```python
from build123d import *

# Parameters (mm, degrees)
SKETCH5_W           = 20
SKETCH5_H           = 20
BOSS_EXTRUDE1_DEPTH = 40
SKETCH7_W           = 12
SKETCH7_H           = 5.480254557
CUT_EXTRUDE3_DEPTH  = 20
SKETCH8_W           = 10
SKETCH8_H           = 10
CUT_EXTRUDE5_DEPTH  = 20
SKETCH12_R          = 3
CUT_EXTRUDE9_DEPTH  = 20
SKETCH16_R          = 4
CUT_EXTRUDE10_DEPTH = 2.5
CUT_EXTRUDE11_START = -2.5
SKETCH17_R          = 4
CUT_EXTRUDE11_DEPTH = 2.5
FILLET8_R           = 8
SKETCH18_R          = 6.023611462
BOSS_EXTRUDE2_DEPTH = 3
SKETCH19_R          = 4
CUT_EXTRUDE12_DEPTH = 10


with BuildPart() as part:
    # Sketch5 → Boss-Extrude1 (new body)
    with BuildSketch(Plane.XY):
        with Locations((0.782482396, -0.960509114)):
            Rectangle(SKETCH5_W, SKETCH5_H)
    extrude(amount=BOSS_EXTRUDE1_DEPTH)

    # Sketch7 → Cut-Extrude3 (cut)
    with BuildSketch(Plane(origin=(10.782482396, 0, 0), x_dir=(0, 0, -1), z_dir=(1, 0, 0))):
        Polygon((-40, 9.039490886), (-40, -0.960509114), (-22, 9.039490886), align=None)
        with Locations((-16, -8.220381835)):
            Rectangle(SKETCH7_W, SKETCH7_H)
        Polygon((-10, 9.039490886), (0, -2.740127279), (0, 9.039490886), align=None)
    extrude(amount=-CUT_EXTRUDE3_DEPTH, mode=Mode.SUBTRACT)

    # Sketch8 → Cut-Extrude5 (cut)
    with BuildSketch(Plane.XZ.offset(10.960509114)):
        with BuildLine():
            Line((-9.217517604, 0), (0.78248238, 0))
            ThreePointArc((0.78248238, 0), (-6.288585421, 2.928932194), (-9.217517604, 10))
            Line((-9.217517604, 10), (-9.217517604, 0))
        make_face()
        with BuildLine():
            Line((10.782482396, 0), (10.782482396, 10))
            ThreePointArc((10.782482396, 10), (7.853550202, 2.928932182), (0.78248238, 0))
            Line((0.78248238, 0), (10.782482396, 0))
        make_face()
        with Locations((0.782482396, 35)):
            Rectangle(SKETCH8_W, SKETCH8_H)
    extrude(amount=-CUT_EXTRUDE5_DEPTH, mode=Mode.SUBTRACT)

    # Sketch10 → Cut-Revolve2 (revolve, cut)
    with BuildSketch(Plane(origin=(0, 9.039490886, 0), x_dir=(1, 0, 0), z_dir=(0, 1, 0))):
        with BuildLine():
            Line((-5.217517604, -16), (6.782482396, -16))
            ThreePointArc((6.782482396, -16), (0.782482396, -22), (-5.217517604, -16))
        make_face()
    revolve(axis=Axis((-5.217517604, 9.039490886, 16), (1, 0, 0)), mode=Mode.SUBTRACT)

    # Sketch12 → Cut-Extrude9 (cut)
    with BuildSketch(Plane(origin=(10.782482396, 0, 0), x_dir=(0, 0, -1), z_dir=(1, 0, 0))):
        with Locations(Location((-35, -5.960509114, 0), (0, 0, 90))):
            Circle(SKETCH12_R)
    extrude(amount=-CUT_EXTRUDE9_DEPTH, mode=Mode.SUBTRACT)

    # Sketch16 → Cut-Extrude10 (cut)
    with BuildSketch(Plane(origin=(10.782482396, 0, 0), x_dir=(0, 0, -1), z_dir=(1, 0, 0))):
        with Locations(Location((-35, -5.960509114, 0), (0, 0, 90))):
            Circle(SKETCH16_R)
    extrude(amount=-CUT_EXTRUDE10_DEPTH, mode=Mode.SUBTRACT)

    # Sketch17 → Cut-Extrude11 (cut)
    with BuildSketch(Plane.ZY.offset(9.217517604).offset(CUT_EXTRUDE11_START)):
        with Locations(Location((35, -5.960509114, 0), (0, 0, 90))):
            Circle(SKETCH17_R)
    extrude(amount=CUT_EXTRUDE11_DEPTH, mode=Mode.SUBTRACT)

    # Fillet8
    fillet8_edges = [part.edges().sort_by_distance(p)[0] for p in [
        (-6.717517604, -0.960509114, 40),
        (8.282482396, -0.960509114, 40),
    ]]
    fillet(fillet8_edges, radius=FILLET8_R)

    # Sketch18 → Boss-Extrude2 (add)
    with BuildSketch(Plane(origin=(0, -5.480254557, 0), x_dir=(-1, 0, 0), z_dir=(0, -1, 0))):
        with Locations((-0.782482396, -16)):
            Circle(SKETCH18_R)
    extrude(amount=BOSS_EXTRUDE2_DEPTH)

    # Sketch19 → Cut-Extrude12 (cut)
    with BuildSketch(Plane(origin=(0, -8.480254557, 0), x_dir=(-1, 0, 0), z_dir=(0, -1, 0))):
        with Locations(Location((-0.782482396, -16, 0), (0, 0, 180))):
            Circle(SKETCH19_R)
    extrude(amount=-CUT_EXTRUDE12_DEPTH, mode=Mode.SUBTRACT)


solid = part.part
```
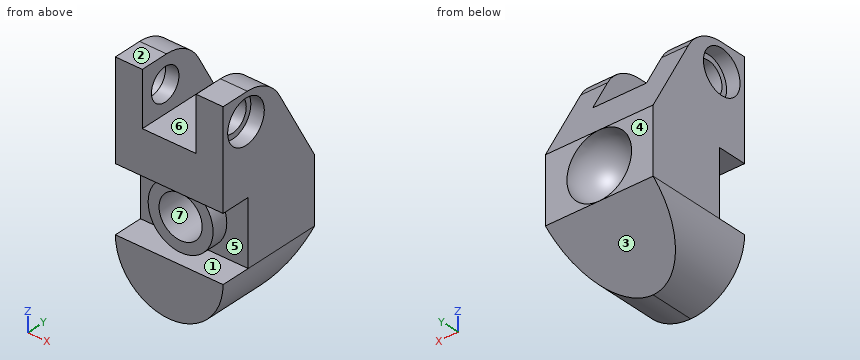
Here's how the part is built. I have some questions about the finished solid (model axes, mm). Face numbers are marked on the shaded views. A direction names the side the tool comes from. Give positions to 0.01 mm unless a question says otherwise; leave off trailing zeros. Loops run counter-clockwise (first coordinate to the right, second up) from the corner with the lowest first, then second, coordinate; pieces in that order, holes last. Notation, with made-up numbers: M 28.5,51 L 54.5,51 A25 ccw 54.5,81 Z; hole C -11.75,33.5 d1. An arc over 180 degrees is marked long. Put each result on its own line as item: value. Start each with the question number.
(1) I want a section at D-D on z = 16. Please give me the cut outline in (x, y), then the cut area to 3 significant figures.
(2) I want a section at B-B on y = 6.5. Please give me the cut outline in (x, z), then the cut area to 3 significant figures.
(3) I want a section at A-A on x = 7.25. Please give me the cut outline in (y, z).
(4) I need wall thicknesses on line 1 along X through (y, z) = (-1.75, 32.5); line 2 along X through (y, z) = (5, 12.5); line 3 along Y through (x, z) = (-4.25, 30). Which ranges of each line are inside material? Lowest first, please. Write a range as [from, to].
(5) If we mould it in two halves opening along Z, with no side actions, what happens to the marked faces 1, 2, 3 and 4? For each: +Z half, -Z half, draft (parallel to the pull), parting line (faces both ways), or undercut.
(6) I want a section at C-C on z = 35. Please give me the cut outline in (x, y), then the cut area to 3 significant figures.
(7) Will these pins go through, and if not, where does the flat tip stop? pin 1 Ø5.5 at (y, z) = (-5.96, 35) entering from +X; pin 2 Ø7 at (x, z) = (0.78, 16) entering from -Y; pin 3 Ø6.5 at (x, z) = (0.5, 17.5) entering from -Y; pin 4 Ø2 at (x, y) = (0.5, 4) entering from -Z.
(8) For the marked faces 5, 6 and 7, which set-ups out of +Z, -Z, +X, -X, +Y, -Y let a thin tool reach every point of the face, with its end or its side?
Answer block:
1. outline: M -9.22,-5.48 L -5.24,-5.48 L -5.24,-8.48 L -3.22,-8.48 L -3.22,1.52 L 4.78,1.52 L 4.78,-8.48 L 6.81,-8.48 L 6.81,-5.48 L 10.78,-5.48 L 10.78,9.04 L 6.78,9.04 A6 cw -5.22,9.04 L -9.22,9.04 Z
1. area: 190 mm^2
2. outline: M -9.22,10 A10 ccw -8.98,7.84 L 10.55,7.84 A10 ccw 10.78,10 L 10.78,26.57 L -9.22,26.57 Z; hole C 0.78,16 d10.87
2. area: 281 mm^2
3. outline: M -10.96,2.37 L 0.06,2.37 L 9.04,10 L 9.04,22 L 1.33,35.89 A8 ccw -5.67,40 L -10.96,40 L -10.96,22 L -5.48,22 L -5.48,10 L -10.96,10 Z; hole C -5.96,35 d6
4. line 1: [-9.22, -4.22], [5.78, 10.78]
4. line 2: [-9.22, -1.94], [3.51, 10.78]
4. line 3: [-10.96, 4.6]
5. face 1: undercut
5. face 2: +Z half
5. face 3: -Z half
5. face 4: draft
6. outline: M -9.22,-10.96 L -4.22,-10.96 L -4.22,-8.96 L -6.72,-8.96 L -6.72,-9.96 L -9.22,-9.96 Z; M -9.22,-1.96 L -6.72,-1.96 L -6.72,-2.96 L -4.22,-2.96 L -4.22,1.82 L -9.22,1.82 Z; M 5.78,-10.96 L 10.78,-10.96 L 10.78,-9.96 L 8.28,-9.96 L 8.28,-8.96 L 5.78,-8.96 Z; M 5.78,-2.96 L 8.28,-2.96 L 8.28,-1.96 L 10.78,-1.96 L 10.78,1.82 L 5.78,1.82 Z
6. area: 57.8 mm^2
7. pin 1: through
7. pin 2: y = 1.52
7. pin 3: y = -8.48
7. pin 4: z = 4.87
8. face 5: +X, -Y
8. face 6: +Z, +Y, -Y
8. face 7: -Y
